```python
from build123d import *

# Parameters (mm, degrees)
SKETCH_1_W            = 20
SKETCH_1_H            = 338
EXTRUDE_1_DEPTH       = 20
EXTRUDE_1_2_DEPTH     = 20
SKETCH_2_W            = 20
SKETCH_2_H            = 20
EXTRUDE_2_DEPTH       = 157
EXTRUDE_4_DEPTH       = 5
SKETCH_6_R            = 22.5
EXTRUDE_5_DEPTH       = 58
EXTRUDE_6_DEPTH       = 15
EXTRUDE_6_DEPTH_BACK  = 350
SKETCH_7_W            = 15
SKETCH_7_H            = 15
SKETCH_12_W           = 20
SKETCH_12_H           = 20
EXTRUDE_10_DEPTH      = 150
SKETCH_13_W           = 20
SKETCH_13_H           = 20
EXTRUDE_11_DEPTH      = 134
SKETCH_14_W           = 20
SKETCH_14_H           = 20
EXTRUDE_12_DEPTH      = 134
EXTRUDE_13_DEPTH      = 15
EXTRUDE_13_DEPTH_BACK = 350
SKETCH_15_W           = 15
SKETCH_15_H           = 15
SKETCH_19_W           = 80
SKETCH_19_H           = 5
EXTRUDE_15_DEPTH      = 100
SKETCH_20_R           = 15
CUT_EXTRUDE_1_DEPTH   = 5


with BuildPart() as part:
    # Sketch 1 → Extrude 1 (new body)
    with BuildSketch(Plane(origin=(0, 0, 0), x_dir=(1, 0, 0), z_dir=(0, 1, 0))):
        with Locations((10, 169)):
            Rectangle(SKETCH_1_W, SKETCH_1_H)
    extrude(amount=EXTRUDE_1_DEPTH)



with BuildPart() as body_2:
    # Sketch 1 → Extrude 1 2 (new body)
    with BuildSketch(Plane(origin=(0, 0, 0), x_dir=(1, 0, 0), z_dir=(0, 1, 0))):
        with Locations((190, 169)):
            Rectangle(SKETCH_1_W, SKETCH_1_H)
    extrude(amount=EXTRUDE_1_2_DEPTH)


with BuildPart() as part_1:
    add(part.part)

    add(body_2.part)  # Extrude 2 merges body 2
    # Sketch 2 → Extrude 2 (add)
    with BuildSketch(Plane(origin=(0, 20, 0), x_dir=(1, 0, 0), z_dir=(0, 1, 0))):
        with Locations((10, 328)):
            Rectangle(SKETCH_2_W, SKETCH_2_H)
        with Locations((190, 328)):
            Rectangle(SKETCH_2_W, SKETCH_2_H)
        with Locations((190, 10)):
            Rectangle(SKETCH_2_W, SKETCH_2_H)
        with Locations((10, 10)):
            Rectangle(SKETCH_2_W, SKETCH_2_H)
    extrude(amount=EXTRUDE_2_DEPTH)

    # Sketch 5 → Extrude 4 (add)
    with BuildSketch(Plane(origin=(0, 177, 0), x_dir=(1, 0, 0), z_dir=(0, 1, 0))):
        with BuildLine():
            Line((0, 0), (200, 0))
            Line((200, 0), (200, 40))
            Line((200, 40), (130, 40))
            Line((130, 40), (130, 60))
            ThreePointArc((130, 60), (100, 90), (70, 60))
            Line((70, 60), (70, 40))
            Line((70, 40), (0, 40))
            Line((0, 40), (0, 0))
        make_face()
        with BuildLine():
            Line((0, 338), (200, 338))
            Line((200, 338), (200, 298))
            Line((200, 298), (130, 298))
            Line((130, 298), (130, 278))
            ThreePointArc((130, 278), (100, 248), (70, 278))
            Line((70, 278), (70, 298))
            Line((70, 298), (0, 298))
            Line((0, 298), (0, 338))
        make_face()
    extrude(amount=EXTRUDE_4_DEPTH)

    # Sketch 6 → Extrude 5 (add)
    with BuildSketch(Plane(origin=(0, 177, 0), x_dir=(-1, 0, 0), z_dir=(0, -1, 0))):
        with Locations(Location((-100, 60, 0), (0, 0, 270))):
            Circle(SKETCH_6_R)
        with Locations(Location((-100, 278, 0), (0, 0, 270))):
            Circle(SKETCH_6_R)
    extrude(amount=EXTRUDE_5_DEPTH)

    # Sketch 7 → Extrude 6 (add, two sides: drawn at the far end of the back side and taken through both)
    with BuildSketch(Plane(origin=(200, 0, 0), x_dir=(0, 0, -1), z_dir=(1, 0, 0)).offset(-EXTRUDE_6_DEPTH_BACK)):
        with Locations((126.5, 27.5)):
            Rectangle(SKETCH_7_W, SKETCH_7_H)
        with Locations((211.5, 27.5)):
            Rectangle(SKETCH_7_W, SKETCH_7_H)
    extrude(amount=EXTRUDE_6_DEPTH + EXTRUDE_6_DEPTH_BACK)

    # Sketch 12 → Extrude 10 (add)
    with BuildSketch(Plane(origin=(0, 182, 0), x_dir=(1, 0, 0), z_dir=(0, 1, 0))):
        with Locations((10, 328)):
            Rectangle(SKETCH_12_W, SKETCH_12_H)
        with Locations((190, 328)):
            Rectangle(SKETCH_12_W, SKETCH_12_H)
        with Locations((10, 10)):
            Rectangle(SKETCH_12_W, SKETCH_12_H)
        with Locations((190, 10)):
            Rectangle(SKETCH_12_W, SKETCH_12_H)
    extrude(amount=EXTRUDE_10_DEPTH)

    # Sketch 13 → Extrude 11 (add)
    with BuildSketch(Plane.XY):
        with Locations((190, 342)):
            Rectangle(SKETCH_13_W, SKETCH_13_H)
        with Locations((10, 342)):
            Rectangle(SKETCH_13_W, SKETCH_13_H)
    extrude(amount=-EXTRUDE_11_DEPTH)

    # Sketch 14 → Extrude 12 (add)
    with BuildSketch(Plane(origin=(0, 0, -338), x_dir=(-1, 0, 0), z_dir=(0, 0, -1))):
        with Locations((-190, 342)):
            Rectangle(SKETCH_14_W, SKETCH_14_H)
        with Locations((-10, 342)):
            Rectangle(SKETCH_14_W, SKETCH_14_H)
    extrude(amount=-EXTRUDE_12_DEPTH)

    # Sketch 15 → Extrude 13 (add, two sides: drawn at the far end of the back side and taken through both)
    with BuildSketch(Plane(origin=(200, 0, 0), x_dir=(0, 0, -1), z_dir=(1, 0, 0)).offset(-EXTRUDE_13_DEPTH_BACK)):
        with Locations((126.5, 359.5)):
            Rectangle(SKETCH_15_W, SKETCH_15_H)
        with Locations((211.5, 359.5)):
            Rectangle(SKETCH_15_W, SKETCH_15_H)
    extrude(amount=EXTRUDE_13_DEPTH + EXTRUDE_13_DEPTH_BACK)

    # Sketch 19 → Extrude 15 (add)
    with BuildSketch(Plane(origin=(0, 0, -219), x_dir=(-1, 0, 0), z_dir=(0, 0, -1))):
        with Locations((90, 17.5)):
            Rectangle(SKETCH_19_W, SKETCH_19_H)
    extrude(amount=-EXTRUDE_15_DEPTH)

    # Sketch 20 → Cut-Extrude 1 (cut)
    with BuildSketch(Plane(origin=(0, 20, 0), x_dir=(1, 0, 0), z_dir=(0, 1, 0))):
        with Locations(Location((-90, 169, 0), (0, 0, 180))):
            Circle(SKETCH_20_R)
    extrude(amount=-CUT_EXTRUDE_1_DEPTH, mode=Mode.SUBTRACT)


solid = part_1.part
```
CAD build for the part. Positions are in the model's coordinates, mm. A direction names the side the tool comes from. Round coordinates to 2 decimals unless told otherwise and drop trailing zeros. Loops run counter-clockwise (first coordinate to the right, second up) from the corner with the lowest first, then second, coordinate; pieces in that order, holes last. Notation, with made-up numbers: (-28, 55) - (-4, 55) arc R20 cw to (-4, 85) - close; hole circle Ø10 at (61, 79). An arc over 180 degrees is marked (long way). Return JSON: item names as keys, results as strings. Group by question number.
Q1. Two-plate mould, pull along Z, no slides. Class faces 6 (the face through (10, 256, -20)), 7 (the face through (180, 298, -326)): +Z half, -Z half, draft (parallel to the pull), parting line (faces both ways), or undercut.
Q2. Band-saw the part on C-C on x = 100. Give the number of separate pieces and of enclosed holes in the cut face, plus the area to 3 significant figures.
Q3. Band-saw the part on B-B on y = 29.5. Give the cut face in (x, z), plus the area to 4 significant figures.
Q4. Drill centre lines: line 1 along Y through (x, z) = (16, -230); line 2 along Z through (x, y) = (-33, 23); line 3 along Y through (x, z) = (66, -307.5). Where is each one in solid material? Low to high. Write a range as [from, to].
Q5. Band-saw the part on D-D on y = 326.5. Give the cut face in (x, z).
Q6. Flat gauge pins, fed straight in: pin 1 Ø2 at (x, z) = (8.5, -275) entering from +Y; pin 2 Ø4 at (y, z) = (179.5, -293) entering from -X; pin 3 Ø10.5 at (x, y) = (53, 356) entering from +Z. Where does each tip first touch, or does it go through?
Q7. Tool access for faces 1 (the face through (190, 256, -318)), 2 (the face through (99, 352, -211)), 3 (the face through (207, 352, -126)), 4 (the face through (30, 27, -134)), 5 (the face through (10, 352, -59)): list every direction of +Z, -Z, +X, -X, +Y, -Y with a clear straight run to the whole face (end or side of a thin tool).
Q8. Band-saw the part on A-A on z = -169. Give the cut face in (x, y).
Solutions:
{
 "1": {"face 6": "undercut", "face 7": "draft"},
 "2": {"separate pieces": "6", "enclosed holes": "0", "area": "7,020 mm^2"},
 "3": {"outline": "(-150, -219) - (215, -219) - (215, -204) - (-150, -204) - close; (-150, -134) - (215, -134) - (215, -119) - (-150, -119) - close; (0, -338) - (20, -338) - (20, -318) - (0, -318) - close; (0, -20) - (20, -20) - (20, 0) - (0, 0) - close; (180, -338) - (200, -338) - (200, -318) - (180, -318) - close; (180, -20) - (200, -20) - (200, 0) - (180, 0) - close", "area": "12,550 mm^2"},
 "4": {"line 1": "y = [0, 20], [332, 352]", "line 2": "z = [-219, -204], [-134, -119]", "line 3": "y = [177, 182]"},
 "5": {"outline": "(0, -338) - (20, -338) - (20, -318) - (0, -318) - close; (0, -20) - (20, -20) - (20, 0) - (0, 0) - close; (180, -338) - (200, -338) - (200, -318) - (180, -318) - close; (180, -20) - (200, -20) - (200, 0) - (180, 0) - close"},
 "6": {"pin 1": "stops at y = 352", "pin 2": "stops at x = 70", "pin 3": "stops at z = -119"},
 "7": {"face 1": "+X, -X", "face 2": "+Z, -Z", "face 3": "+Z, -Z, +X", "face 4": "+X, -X, +Y", "face 5": "+Z, +X, -X, +Y"},
 "8": {"outline": "(-130, 15) - (-105, 15) - (-105, 20) - (-130, 20) - close; (-75, 15) - (-50, 15) - (-50, 20) - (-75, 20) - close; (0, 0) - (20, 0) - (20, 20) - (0, 20) - close; (180, 0) - (200, 0) - (200, 20) - (180, 20) - close"}
}
